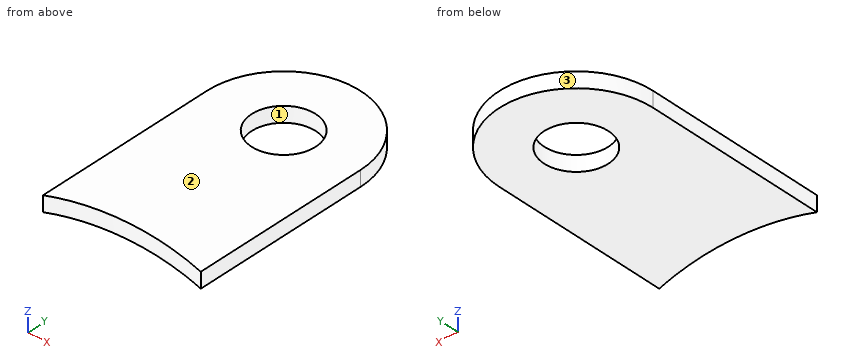
from build123d import *

# Parameters (mm, degrees)
SKETCH1_R            = 7.9375
SKETCH1_R_2          = 3
BOSS_EXTRUDE1_DEPTH  = 1.5875
M6_CLEARANCE_HOLE1_D = 6.6
SKETCH5_W            = 15.875
SKETCH5_H            = 6.35
CUT_EXTRUDE2_DEPTH   = 27.658658303
CUT_EXTRUDE3_DEPTH   = 21.698467637


with BuildPart() as part:
    # Sketch1 → Boss-Extrude1 (new body)
    # profile 1 of 3: a face of its own
    with BuildSketch(Plane.XY):
        Circle(SKETCH1_R)
        Circle(SKETCH1_R_2, mode=Mode.SUBTRACT)
    # profile 2 of 3: a face of its own
    with BuildSketch(Plane.XY):
        with BuildLine():
            ThreePointArc((7.9375, 0), (0, -7.9375), (-7.9375, 0))
            Line((-7.9375, 0), (-7.9375, -25.4))
            Line((-7.9375, -25.4), (7.9375, -25.4))
            Line((7.9375, -25.4), (7.9375, 0))
        make_face()
    # profile 3 of 3: a face of its own
    with BuildSketch(Plane.XY):
        Circle(SKETCH1_R_2)
    extrude(amount=BOSS_EXTRUDE1_DEPTH)

    # M6 Clearance Hole1 (through all)
    with Locations(Plane.XY.offset(1.5875)):
        with Locations((0, 0)):
            Hole(M6_CLEARANCE_HOLE1_D / 2)

    # Sketch5 → Cut-Extrude2 (cut, through all)
    with BuildSketch(Plane.XY.offset(1.5875)):
        with Locations((0, -22.225)):
            Rectangle(SKETCH5_W, SKETCH5_H)
    extrude(amount=-CUT_EXTRUDE2_DEPTH, mode=Mode.SUBTRACT)

    # Sketch6 → Cut-Extrude3 (cut, through all)
    with BuildSketch(Plane(origin=(0, 0, 0), x_dir=(-1, 0, 0), z_dir=(0, 0, -1))):
        with BuildLine():
            add(Edge.make_bspline(
                [(12.030285896, -22.899436183), (1.652467131, 0.283766307), (-38.284264846, -17.593667439), (-27.906446081, -40.776869929), (-17.528627316, -63.960072418), (22.408104661, -46.082638673), (12.030285896, -22.899436183)],
                knots=[0, 0, 0, 0, 0.5, 0.5, 0.5, 1, 1, 1, 1], degree=3, weights=[1, 0.333333333, 0.333333333, 1, 0.333333333, 0.333333333, 1]))
        make_face()
    extrude(amount=-CUT_EXTRUDE3_DEPTH, mode=Mode.SUBTRACT)


solid = part.part
Can you work these out from the model? Positions are in its coordinate system, mm. Face numbers are marked on the shaded views. Round coordinates to 2 decimals unless told otherwise and drop trailing zeros. Write each loop counter-clockwise with the first axis right and the second up, starting at its lowest first coordinate (ties: lowest second). Pieces come first, ordered by that corner, then holes. Notation, with made-up numbers: (44, -34) -> (64, -34) arc R32 ccw to (64, -7) -> close; hole circle Ø1 at (-34.75, 30.25). An arc over 180 degrees is marked (long way). One line per question, with ' | ' between items. Start each with the question number.
1) Suppose I cut it at A-A on y = -0.5. Write out the boundary of the cut face in (x, z), then the cut area to 3 significant figures.
2) If we mould it in two halves opening along X, with no side actions, what happens to the marked faces 1, 2 and 3? For each: released by +X, released by -X, zero draft, split by the parting line, or undercut.
3) I need wall thicknesses on line 1 (Y direction, x = 0, z = 0.6); line 2 (Y direction, x = -2.75, z = 1.2); line 3 (X direction, y = -1, z = 1.2). Which ranges of each line are inside material? Lowest first, please. Write a range as [from, to].
Return value:
1) outline: (-7.94, 0) -> (-3.26, 0) -> (-3.26, 1.59) -> (-7.94, 1.59) -> close; (3.26, 0) -> (7.94, 0) -> (7.94, 1.59) -> (3.26, 1.59) -> close | area: 14.8 mm2
2) face 1: undercut | face 2: zero draft | face 3: split by the parting line
3) line 1: y = [-17.2, -3.3], [3.3, 7.94] | line 2: y = [-17.35, -1.82], [1.82, 7.45] | line 3: x = [-7.94, -3.14], [3.14, 7.94]
